Could you check a few things on this model? Use its own coordinates, in mm. Face numbers are marked on the shaded views. A direction names the side the tool comes from. Coordinates: 2 decimals unless noted, no trailing zeros. Write each loop counter-clockwise with the first axis right and the second up, starting at its lowest first coordinate (ties: lowest second). Pieces come first, ordered by that corner, then holes.
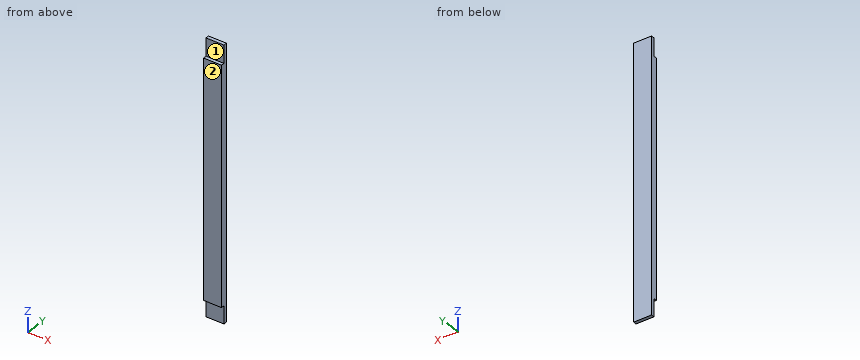
```python
from build123d import *

# Parameters (mm, degrees)
F0_W     = 50.8
F0_H     = 19.05
F1_DEPTH = 774.7
F2_W     = 122.43557321
F2_H     = 50.8
F2_W_2   = 343.1604206562
F3_DEPTH = 25.4


# Not quite as in the source:
# - a feature names something its author has since deleted; it is built from what else it names


with BuildPart() as f1:
    # F0 (on Top) → F1 (new body)
    with BuildSketch(Plane.XY):
        Rectangle(F0_W, F0_H)
    extrude(amount=F1_DEPTH)

    # F2 (on Front) → F3 (cut)
    with BuildSketch(Plane.XZ):
        with Locations((22.4465244144, 25.4)):
            Rectangle(F2_W, F2_H)
        with Locations((-38.7818217278, 749.3)):
            Rectangle(F2_W_2, F2_H)
    extrude(amount=F3_DEPTH, mode=Mode.SUBTRACT)


solid = f1.part
```
Item 1: I want a section at A-A, the plane x = -15.5. List the corners of the cut face in (y, z) for me (3 decimals).
Item 2: Which directions (+Z, -Z, +X, -X, +Y, -Y) give clear straight access to the entire face, cutting with the end or side of a thin tool? Please do the marked faces 1 and 2.
Item 3: Will these pins go through, and if not, where does the flat tip stop? pin 1 Ø3 at (x, y) = (14, -4.5) entering from -Z; pin 2 Ø4 at (x, y) = (-7.5, 7) entering from -Z; pin 3 Ø15 at (x, z) = (9.5, 18.5) entering from -Y.
Item 4: I want a section at B-B, the plane y = -5.25. List the corners of the cut face in (x, z) for me.
Item 5: If I drill on line 1 along Z through (x, y) = (-14, -4); line 2 along Y through (x, z) = (-22, 34.5) (3 decimals), over which ranges is the centre line in solid material (lowest first)?
Taken from the geometry:
1. outline: (-9.525, 50.8) - (0, 50.8) - (0, 0) - (9.525, 0) - (9.525, 774.7) - (0, 774.7) - (0, 723.9) - (-9.525, 723.9) - close
2. face 1: +Z, +X, -X, -Y
2. face 2: +Z, -Z, +X, -X, -Y
3. pin 1: stops at z = 50.8
3. pin 2: stops at z = 0
3. pin 3: stops at y = 0
4. outline: (-25.4, 50.8) - (25.4, 50.8) - (25.4, 723.9) - (-25.4, 723.9) - close
5. line 1: z = 50.8 to 723.9
5. line 2: y = 0 to 9.525
